Autodesk Inventor part; units mm, degrees
ref_plane "YZ Plane" through (0, 0, 0) normal (1, 0, 0) x (0, 1, 0)
ref_plane "XZ Plane" through (0, 0, 0) normal (0, 1, 0) x (-1, 0, 0)
ref_plane "XY Plane" through (0, 0, 0) normal (0, 0, 1) x (1, 0, 0)
ref_plane "Work Plane1" through (153.3626, 3.175, 315.1376) normal (0, 1, 0) x (1, 0, 0)
sketch "Sketch2" plane through (153.3626, 3.175, 315.1376) normal (0, 1, 0) x (1, 0, 0)
  circle A0 centre (-50.8, 212.575) radius 6.35
  line L0 (-50.8, 212.575) -> (-50.8, 187.175)
  line L1 (-50.8, 187.175) -> (-102.9735, 187.175)
  circle A1 centre (-88.9, 139.7) radius 2.65
  circle A2 centre (-88.9, 114.3) radius 2.65
  line L2 (-101.6, 142.5126) -> (-101.6, 66.675)
  line L3 (-50.8, 212.575) -> (-25.4, 212.575)
  line L4 (-25.4, 212.575) -> (-25.4, 238.8185)
  line L5 (-101.6, 142.5126) -> (-101.6, 66.675)
  arc A3 (-88.9, 28.575) -> (-12.7, 28.575) centre (-50.8, 28.575) ccw
  circle A4 centre (-50.8, 28.575) radius 38.1
  line L6 (-101.6, 66.675) -> (-82.55, 66.675)
  line L7 (-82.55, 45.5611) -> (-82.55, 142.5126)
  arc A5 (-76.2, 28.575) -> (-25.4, 28.575) centre (-50.8, 28.575) ccw
  line L8 (-82.55, 66.675) -> (-76.2, 66.675)
  line L9 (-76.2, 34.5626) -> (-76.2, 28.575)
  line L10 (-101.6, 142.5126) -> (-82.55, 142.5126)
  line L11 (-82.55, 40.9126) -> (-82.55, 40.9126)
  arc A6 (-76.2, 34.5626) -> (-79.375, 40.0618) centre (-82.55, 34.5626) ccw
  arc A7 (-82.55, 45.5611) -> (-79.375, 40.0618) centre (-76.2, 45.5611) ccw
  line L12 (-82.55, 142.5126) -> (-82.55, 148.8626)
  line L13 (-76.2, 155.2126) -> (-76.2, 155.2126)
  line L14 (-69.85, 161.5626) -> (-69.85, 187.175)
  arc A8 (-76.2, 155.2126) -> (-69.85, 161.5626) centre (-76.2, 161.5626) ccw
  arc A9 (-76.2, 155.2126) -> (-82.55, 148.8626) centre (-76.2, 148.8626) ccw
  line L15 (-19.05, 45.5611) -> (-19.05, 142.5126)
  line L16 (-25.4, 34.5626) -> (-25.4, 28.575)
  arc A10 (-22.225, 40.0618) -> (-25.4, 34.5626) centre (-19.05, 34.5626) ccw
  arc A11 (-22.225, 40.0618) -> (-19.05, 45.5611) centre (-25.4, 45.5611) ccw
  arc A12 (19.05, 161.775) -> (0, 142.725) centre (19.05, 142.725) ccw
  circle A13 centre (19.05, 142.725) radius 19.05
  circle A14 centre (19.05, 142.725) radius 38.1006
  line L17 (-50.8, 212.575) -> (-25.4, 212.575)
  line L18 (-25.4, 212.575) -> (-25.4, 264.7485)
  circle A15 centre (22.075, 250.675) radius 2.65
  circle A16 centre (47.475, 250.675) radius 2.65
  line L19 (19.2624, 263.375) -> (95.1, 263.375)
  line L20 (-50.8, 212.575) -> (-50.8, 187.175)
  line L21 (19.2624, 263.375) -> (95.1, 263.375)
  arc A17 (133.2, 174.475) -> (133.2, 250.675) centre (133.2, 212.575) ccw
  circle A18 centre (133.2, 212.575) radius 38.1
  line L22 (95.1, 263.375) -> (95.1, 244.325)
  line L23 (116.2139, 244.325) -> (19.2624, 244.325)
  arc A19 (133.2, 187.175) -> (133.2, 237.975) centre (133.2, 212.575) ccw
  line L24 (95.1, 244.325) -> (95.1, 237.975)
  line L25 (127.2124, 237.975) -> (133.2, 237.975)
  line L26 (120.8624, 244.325) -> (120.8624, 244.325)
  arc A20 (121.7132, 241.15) -> (127.2124, 237.975) centre (127.2124, 244.325) ccw
  arc A21 (121.7132, 241.15) -> (116.2139, 244.325) centre (116.2139, 237.975) ccw
  line L27 (19.2624, 244.325) -> (12.9124, 244.325)
  line L28 (6.5624, 237.975) -> (6.5624, 237.975)
  line L29 (0.2124, 231.625) -> (-25.4, 231.625)
  arc A22 (0.2124, 231.625) -> (6.5624, 237.975) centre (0.2124, 237.975) ccw
  arc A23 (12.9124, 244.325) -> (6.5624, 237.975) centre (12.9124, 237.975) ccw
  line L30 (116.2139, 180.825) -> (19.2624, 180.825)
  arc A24 (127.2124, 187.175) -> (121.7132, 184) centre (127.2124, 180.825) ccw
  arc A25 (116.2139, 180.825) -> (121.7132, 184) centre (116.2139, 187.175) ccw
  line L31 (127.2124, 187.175) -> (133.2, 187.175)
  arc A26 (-34.6191, 237.975) -> (4.5675, 256.4477) centre (-34.6191, 288.775) ccw
  arc A27 (-25.4, 238.8185) -> (4.5675, 256.4477) centre (-34.6191, 288.775) ccw
  arc A28 (19.2624, 263.375) -> (4.5675, 256.4477) centre (19.2624, 244.325) ccw
  arc A29 (19.2624, 263.375) -> (4.5675, 256.4477) centre (19.2624, 244.325) ccw
  line L32 (0, 66.675) -> (0, 142.725)
  line L33 (0, 142.725) -> (0, 25.7278)
  arc A30 (-94.6727, 157.2075) -> (-101.6, 142.5126) centre (-82.55, 142.5126) ccw
  arc A31 (-94.6727, 157.2075) -> (-101.6, 142.5126) centre (-82.55, 142.5126) ccw
  arc A32 (-94.6727, 157.2075) -> (-76.2, 196.3941) centre (-127, 196.3941) ccw
  arc A33 (-94.6727, 157.2075) -> (-76.2, 196.3941) centre (-127, 196.3941) ccw
  line L34 (19.05, 161.775) -> (95.1, 161.775)
  line L35 (-101.6, 66.675) -> (-101.6, 47.625) construction
  line L36 (-101.6, 47.625) -> (-88.9, 47.625) construction
  line L37 (-88.9, 47.625) -> (-88.9, 28.575) construction
  spline S0 degree 3 poles (-101.6, 66.675) (-101.6, 47.625) (-88.9, 47.625) (-88.9, 28.575) knots 1 1 1 1 2 2 2 2
  line L38 (-50.8, 28.575) -> (-50.8, 60.9646)
  spline S1 degree 3 poles (0, 66.675) (0, 47.625) (-12.7, 47.625) (-12.7, 28.575) knots 1 1 1 1 2 2 2 2
  line L39 (0, 66.675) -> (0, 47.625) construction
  line L40 (0, 47.625) -> (-12.7, 47.625) construction
  line L41 (-12.7, 47.625) -> (-12.7, 28.575) construction
  spline S2 degree 3 poles (95.1, 263.375) (114.15, 263.375) (114.15, 250.675) (133.2, 250.675) knots 1 1 1 1 2 2 2 2
  line L42 (95.1, 263.375) -> (114.15, 263.375) construction
  line L43 (114.15, 263.375) -> (114.15, 250.675) construction
  line L44 (114.15, 250.675) -> (133.2, 250.675) construction
  spline S3 degree 3 poles (95.1, 161.775) (114.15, 161.775) (114.15, 174.475) (133.2, 174.475) knots 1 1 1 1 2 2 2 2
  line L45 (95.1, 161.775) -> (114.15, 161.775) construction
  line L46 (114.15, 161.775) -> (114.15, 174.475) construction
  line L47 (114.15, 174.475) -> (133.2, 174.475) construction
  circle A34 centre (-88.9, 88.9) radius 2.65
  circle A35 centre (-88.9, 88.9) radius 2.65
  circle A36 centre (-88.9, 63.5) radius 2.65
  circle A37 centre (-88.9, 63.5) radius 2.65
  circle A38 centre (-82.55, 28.575) radius 2.65
  circle A39 centre (-82.55, 28.575) radius 2.65
  circle A40 centre (-19.05, 28.575) radius 2.65
  circle A41 centre (-19.05, 28.575) radius 2.65
  circle A42 centre (-12.7, 63.5) radius 2.65
  circle A43 centre (-12.7, 63.5) radius 2.65
  circle A44 centre (-12.7, 88.9) radius 2.65
  circle A45 centre (-12.7, 88.9) radius 2.65
  circle A46 centre (-12.7, 114.3) radius 2.65
  circle A47 centre (-12.7, 114.3) radius 2.65
  circle A48 centre (-12.7, 139.7) radius 2.65
  circle A49 centre (-12.7, 139.7) radius 2.65
  circle A50 centre (22.075, 174.475) radius 2.65
  circle A51 centre (22.075, 174.475) radius 2.65
  circle A52 centre (47.475, 174.475) radius 2.65
  circle A53 centre (47.475, 174.475) radius 2.65
  circle A54 centre (72.875, 174.475) radius 2.65
  circle A55 centre (72.875, 174.475) radius 2.65
  circle A56 centre (98.275, 174.475) radius 2.65
  circle A57 centre (98.275, 174.475) radius 2.65
  circle A58 centre (133.2, 180.825) radius 2.65
  circle A59 centre (133.2, 180.825) radius 2.65
  circle A60 centre (133.2, 244.325) radius 2.65
  circle A61 centre (133.2, 244.325) radius 2.65
  circle A62 centre (98.275, 250.675) radius 2.65
  circle A63 centre (98.275, 250.675) radius 2.65
  circle A64 centre (72.875, 250.675) radius 2.65
  point P0 (-153.3626, 315.1376)
  point P1 (-82.55, 155.2126)
  point P2 (-69.85, 155.2126)
  point P3 (6.5624, 244.325)
  point P4 (6.5624, 231.625)
  point P5 (-77.0435, 187.175)
  point P6 (-88.9, 28.575)
  point P7 (-12.7, 28.575)
  point P8 (133.2, 174.475)
  point P9 (133.2, 250.675)
  point P10 (-25.4, 238.8185)
  point P11 (6.5624, 237.975)
  point P12 (19.2624, 244.325)
  dimension "d40" = 25.4
  dimension "d43" = 19.05
  dimension "d46" = 12.7
  dimension "d47" = 76.2
  dimension "d48" = 101.6
  dimension "d49" = 6.35
  dimension "d50" = 12.7
  dimension "d51" = 12.7
  dimension "d52" = 6.35
  dimension "d53" = 19.05
  dimension "d54" = 19.05
extrude "Extrusion2" add sketch "Sketch2" along normal blind 32.004 contours L4 A26 A28 L19 L22 L23 L27 A23 A22 L29 | L14 A8 A9 L12 L10 A30 A32 L1 | L10 L7 L6 L2 | S2 A18 L23 L22 | L6 L7 A4 S0 | A17 A18 L30 A25 A24 L31 A19 L25 A20 A21 L23 | A4 L7 A7 A6 L9 A5 L16 A10 A11 L15 A3 | A4 L15 A14 L32 S1 | A18 S3 L34 A14 L30 | A14 L34 A12 L32
properties part number "Gearbox Cover Large"
Verification items for the finished model (mm, model axes). A direction names the side the tool comes from. Give positions to 0.01 mm unless a question says otherwise; leave off trailing zeros. Order: outer loops, then holes, each group sorted by start corner. A loop starts at its lowest first (then second) coordinate and runs counter-clockwise, first axis right, second up. Notation, with made-up numbers: M 64.25,82.5 L 108.25,82.5 A17 cw 108.25,87.5 Z; hole C 60,58 d2. An arc over 180 degrees is marked long. Return JSON: item names as keys, results as strings. Group by question number.
1) Scan lines: line 1 (X direction, y = 10.5, z = 201); line 2 (X direction, y = 31.5, z = 193); line 3 (Z direction, x = 251.5, y = 16). Record each from-to range of solid material in increasing order.
2) Section check C-C on y = 14. Give the number of separate pieces and of enclosed holes in the cut face, and give its area (3 significant figures).
3) Mould release check, pull along X, two halves, no side actions. Record for faces 5 (the face through (145.175, 18.953, 145.771)), 6 (the face through (147, 3.175, 167)), 7 (the face through (158.795, 18.953, 159.091)): pulls with the +X half, pulls with the -X half, needs draft (parallel to the pull), parting line crosses it, or undercut.
4) Section check D-D on z = 99.5. Record the cut outline in (x, y) (3 decimals).
5) Access from +Z, -Z, +X, -X, +Y, -Y to the whole of each face (thin tool, end or side, straight path). Record for faces 1 (the face through (153.363, 19, 211)), 2 (the face through (219, 19, 70.813)), 3 (the face through (284, 19, 127.963)), 4 (the face through (80, 19, 127.963)).
6) Section check A-A on x = 236. Record the cut outline in (y, z) (3 decimals).
7) Go/stop test with flat-tipped pins: pin 1 Ø9.5 at (x, y) = (238.5, 22) entering from +Z; pin 2 Ø6 at (y, z) = (16, 78.5) entering from -X; pin 3 Ø4 at (x, z) = (286.56, 134.31) entering from +Y; pin 4 Ø10 at (y, z) = (10.5, 292.5) entering from -X. Record where each tip stops, or that it passes through.
8) Section check B-B on z = 188.5. Record the cut outline in (x, y) (3 decimals), and give its area (3 significant figures).
Answer block:
{
 "1": {"line 1": "x = 51.76 to 61.82, 67.11 to 70.81, 134.31 to 138.02, 143.31 to 153.36", "line 2": "x = 51.76 to 70.81, 134.31 to 153.36", "line 3": "z = 51.88 to 61.82, 67.11 to 70.81, 134.31 to 138.02, 143.31 to 153.25"},
 "2": {"separate pieces": "1", "enclosed holes": "20", "area": "12,300 mm^2"},
 "3": {"face 5": "undercut", "face 6": "needs draft", "face 7": "pulls with the +X half"},
 "4": {"outline": "M 311.777,3.175 L 324.539,3.175 L 324.539,35.179 L 311.777,35.179 Z"},
 "5": {"face 1": "+Z, +X, +Y, -Y", "face 2": "+Y, -Y", "face 3": "-X, +Y, -Y", "face 4": "-Z, -X, +Y, -Y"},
 "6": {"outline": "M 3.175,51.763 L 35.179,51.763 L 35.179,70.813 L 3.175,70.813 Z; M 3.175,134.313 L 35.179,134.313 L 35.179,153.363 L 3.175,153.363 Z"},
 "7": {"pin 1": "stops at z = 153.36", "pin 2": "stops at x = 127.96", "pin 3": "passes through", "pin 4": "stops at x = 64.47"},
 "8": {"outline": "M 51.763,3.175 L 70.813,3.175 L 70.813,35.179 L 51.763,35.179 Z; M 134.313,3.175 L 153.363,3.175 L 153.363,35.179 L 134.313,35.179 Z", "area": "1,220 mm^2"}
}
